The model under review builds one solid part; all positions refer to its coordinate system, in mm. Round coordinates to 2 decimals unless told otherwise and drop trailing zeros. Write each loop counter-clockwise with the first axis right and the second up, starting at its lowest first coordinate (ties: lowest second). Pieces come first, ordered by that corner, then holes. Notation, with made-up numbers: (85, -37.5) -> (111, -37.5) arc R11 cw to (111, -18.5) -> close; hole circle Ø9 at (-13, -31.75). An arc over 180 degrees is marked (long way). Answer in a Markdown table with one row per item. Add a question column.
```python
from build123d import *

# Parameters (mm, degrees)
BOSS_EXTRUDE1_DEPTH = 30
CUT_EXTRUDE1_DEPTH  = 31


with BuildPart() as part:
    # Sketch1 → Boss-Extrude1 (new body)
    with BuildSketch(Plane(origin=(0, 0, 0), x_dir=(1, 0, 0), z_dir=(0, 1, 0))):
        Polygon((0, 0), (0, 32), (32, 0), align=None)
    extrude(amount=BOSS_EXTRUDE1_DEPTH)

    # Sketch2 → Cut-Extrude1 (cut, through all)
    with BuildSketch(Plane(origin=(0, 30, 0), x_dir=(1, 0, 0), z_dir=(0, 1, 0))):
        Polygon((0, 27), (5, 27), (0, 32), align=None)
        Polygon((27, 0), (32, 0), (27, 5), align=None)
    extrude(amount=-CUT_EXTRUDE1_DEPTH, mode=Mode.SUBTRACT)


solid = part.part
```
1. For L1, parallel to Z at x = 13.25, y = 17; L2, parallel to X at y = 15, z = -8; L3, parallel to X at y = 7.5, z = -9.5, list the stretches that pass through material, from the lowest coordinate up.
2. Insertion check: pin 1 Ø10 at (x, y) = (17.5, 23.5) entering from -Z; pin 2 Ø1 at (x, y) = (6.5, 4) entering from -Z. Each pin has a flat end and moves straight along its axis. Give the tip position at first contact, or say it passes through.
3. Add section A-A on y = 20.75. Write out the cut boundary in (x, z).
4. Add section C-C on z = -6.5. Write out the cut boundary in (x, y).
5. Add section B-B on x = 7.25. Write out the cut boundary in (y, z), plus the area to 4 significant figures.
Filled in:
| question | item | result |
|---|---|---|
| 1 | L1 | -18.75 to 0 |
| 1 | L2 | 0 to 24 |
| 1 | L3 | 0 to 22.5 |
| 2 | pin 1 | z = -19.5 |
| 2 | pin 2 | z = -26 |
| 3 | outline | (0, -27) -> (5, -27) -> (27, -5) -> (27, 0) -> (0, 0) -> close |
| 4 | outline | (0, 0) -> (25.5, 0) -> (25.5, 30) -> (0, 30) -> close |
| 5 | outline | (0, -24.75) -> (30, -24.75) -> (30, 0) -> (0, 0) -> close |
| 5 | area | 742.5 mm² |
